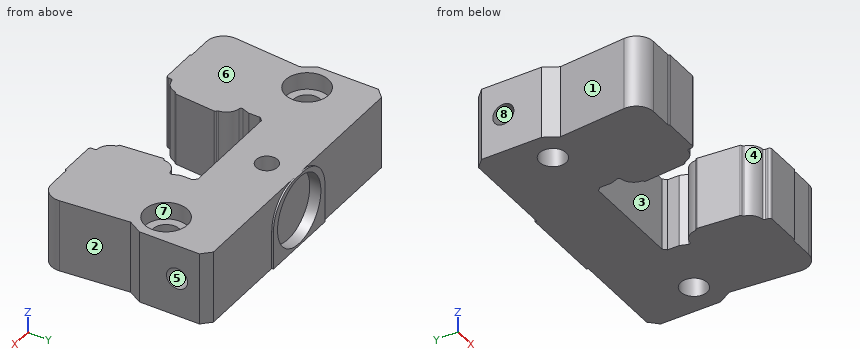
```python
from build123d import *

# Parameters (mm, degrees)
EXTRUDE1_DEPTH                          = 4.25
CBORE_FOR_M5_HEX_HEAD_BOLT2_D           = 3.1
CBORE_FOR_M5_HEX_HEAD_BOLT2_CBORE_D     = 5
CBORE_FOR_M5_HEX_HEAD_BOLT2_CBORE_DEPTH = 2
F_2_5_2_5_DIAMETER_HOLE1_D              = 2.5
F_2_5_2_5_DIAMETER_HOLE1_DEPTH          = 6
F_2_5_2_5_DIAMETER_HOLE1_TIP            = 0.751075774
SKETCH13_R                              = 4
EXTRUDE3_DEPTH                          = 0.2
CUT_EXTRUDE2_START                      = -1.3
SKETCH15_R                              = 4
CUT_EXTRUDE2_DEPTH                      = 1.3
FILLET1_R                               = 0.3
SKETCH16_W                              = 4.5
SKETCH16_H                              = 1.23


with BuildPart() as part:
    # Sketch1 → Extrude1 (new, symmetric)
    with BuildSketch(Plane.XY):
        with BuildLine():
            Line((4.92550995, -3.000896773), (5.340282634, -7.741770244))
            ThreePointArc((5.340282634, -7.741770244), (5.387571197, -7.845597639), (5.489639003, -7.896573115))
            ThreePointArc((5.489639003, -7.896573115), (5.583252131, -7.939368417), (5.635340188, -8.028147299))
            ThreePointArc((5.635340188, -8.028147299), (6.141739158, -8.88598399), (7.051010463, -9.292861611))
            ThreePointArc((7.051010463, -9.292861611), (7.196097182, -9.367838396), (7.25433228, -9.520417385))
            Line((7.25433228, -9.520417385), (7.25433228, -10.089549749))
            Line((7.25433228, -10.089549749), (11.66333313, -10.10000765))
            Line((11.66333313, -10.10000765), (11.81333313, -9.95000765))
            Line((11.81333313, -9.95000765), (14.47525163, -9.95000765))
            ThreePointArc((14.47525163, -9.95000765), (15.889465188, -9.36422121), (16.475251623, -7.95000765))
            ThreePointArc((16.475251623, -7.95000765), (16.473348066, -7.862768875), (16.467641019, -7.775696164))
            Line((16.467641019, -7.775696164), (15.777924964, 0.107794413))
            Line((15.777924964, 0.107794413), (16.697189707, 1.700007653))
            Line((16.697189707, 1.700007653), (16.697189707, 8.700007649))
            Line((16.697189707, 8.700007649), (15.697189707, 9.70000765))
            Line((15.697189707, 9.70000765), (-15.302810298, 9.70000765))
            Line((-15.302810298, 9.70000765), (-16.302810293, 8.700007655))
            Line((-16.302810293, 8.700007655), (-16.302810293, 1.70000765))
            Line((-16.302810293, 1.70000765), (-15.383545551, 0.107794412))
            Line((-15.383545551, 0.107794412), (-16.073261605, -7.775696165))
            ThreePointArc((-16.073261605, -7.775696165), (-15.555426882, -9.301188065), (-14.080872208, -9.95000765))
            Line((-14.080872208, -9.95000765), (-11.418953708, -9.95000765))
            Line((-11.418953708, -9.95000765), (-11.268953705, -10.10000765))
            Line((-11.268953705, -10.10000765), (-6.85995286, -10.089549753))
            Line((-6.85995286, -10.089549753), (-6.85995286, -9.520417385))
            ThreePointArc((-6.85995286, -9.520417385), (-6.801717763, -9.367838396), (-6.656631044, -9.292861611))
            ThreePointArc((-6.656631044, -9.292861611), (-5.747359739, -8.885983989), (-5.240960769, -8.028147299))
            ThreePointArc((-5.240960769, -8.028147299), (-5.188872711, -7.939368417), (-5.095259583, -7.896573115))
            ThreePointArc((-5.095259583, -7.896573115), (-4.993191778, -7.845597639), (-4.945903214, -7.741770244))
            Line((-4.945903214, -7.741770244), (-4.531130531, -3.000896773))
            ThreePointArc((-4.531130531, -3.000896773), (-4.530642578, -2.993452056), (-4.530479824, -2.985993141))
            ThreePointArc((-4.530479824, -2.985993141), (-4.563077813, -2.885564642), (-4.648443372, -2.823425817))
            ThreePointArc((-4.648443372, -2.823425817), (-4.731098063, -2.76492056), (-4.766166593, -2.669921291))
            ThreePointArc((-4.766166593, -2.669921291), (-5.198040021, -1.644927498), (-6.18433448, -1.130777545))
            ThreePointArc((-6.18433448, -1.130777545), (-6.349566009, -1.022272522), (-6.368749921, -0.825532146))
            Line((-6.368749921, -0.825532146), (-6.070902174, -0.007202189))
            ThreePointArc((-6.070902174, -0.007202189), (-6.057367635, 0.043309401), (-6.05280996, 0.095403855))
            Line((-6.05280996, 0.095403855), (-6.05280996, 1.399955293))
            Line((-6.05280996, 1.399955293), (-5.652810289, 1.800007648))
            Line((-5.652810289, 1.800007648), (6.047189708, 1.800007648))
            Line((6.047189708, 1.800007648), (6.44718938, 1.399955292))
            Line((6.44718938, 1.399955292), (6.44718938, 0.095403855))
            ThreePointArc((6.44718938, 0.095403855), (6.451747054, 0.043309401), (6.465281594, -0.007202188))
            Line((6.465281594, -0.007202188), (6.763129341, -0.825532146))
            ThreePointArc((6.763129341, -0.825532146), (6.773460706, -0.864089327), (6.77693973, -0.903854759))
            ThreePointArc((6.77693973, -0.903854759), (6.720404632, -1.054509523), (6.578713899, -1.130777545))
            ThreePointArc((6.578713899, -1.130777545), (5.59241944, -1.644927498), (5.160546013, -2.669921291))
            ThreePointArc((5.160546013, -2.669921291), (5.125477483, -2.76492056), (5.042822792, -2.823425817))
            ThreePointArc((5.042822792, -2.823425817), (4.953208331, -2.891697239), (4.92550995, -3.000896773))
        make_face()
    extrude(amount=EXTRUDE1_DEPTH, both=True)

    # CBORE for M5 Hex Head Bolt2 (through all)
    with Locations(Plane(origin=(-12.802810293, 2.596389855, 4.25), x_dir=(1, 0, 0), z_dir=(0, 0, 1))):
        with Locations((0, 0), (26, 0)):
            CounterBoreHole(CBORE_FOR_M5_HEX_HEAD_BOLT2_D / 2, CBORE_FOR_M5_HEX_HEAD_BOLT2_CBORE_D / 2, CBORE_FOR_M5_HEX_HEAD_BOLT2_CBORE_DEPTH)

    # Ø2.5 (2.5) Diameter Hole1
    with Locations(Plane(origin=(0.197189707, 6.127234967, 4.25), x_dir=(1, 0, 0), z_dir=(0, 0, 1))):
        with Locations((0, 0)):
            Hole(F_2_5_2_5_DIAMETER_HOLE1_D / 2, depth=F_2_5_2_5_DIAMETER_HOLE1_DEPTH)
            with Locations((0, 0, -(F_2_5_2_5_DIAMETER_HOLE1_DEPTH + F_2_5_2_5_DIAMETER_HOLE1_TIP / 2))):  # 118° drill point
                Cone(0, F_2_5_2_5_DIAMETER_HOLE1_D / 2, F_2_5_2_5_DIAMETER_HOLE1_TIP, mode=Mode.SUBTRACT)

    # Sketch13 → Extrude3 (add)
    with BuildSketch(Plane(origin=(0, 9.70000765, 0), x_dir=(1, 0, 0), z_dir=(0, 1, 0))):
        with BuildLine():
            Line((-4.552810293, 4.25), (-4.552810293, -0.25))
            ThreePointArc((-4.552810293, -0.25), (-3.381237418, -3.078427125), (-0.552810293, -4.25))
            Line((-0.552810293, -4.25), (0.947189707, -4.25))
            ThreePointArc((0.947189707, -4.25), (3.775616832, -3.078427125), (4.947189707, -0.25))
            Line((4.947189707, -0.25), (4.947189707, 4.25))
            Line((4.947189707, 4.25), (-4.552810293, 4.25))
        make_face()
        with Locations(Location((0.197189707, 0, 0), (0, 0, 270))):
            Circle(SKETCH13_R, mode=Mode.SUBTRACT)
    extrude(amount=EXTRUDE3_DEPTH)

    # Sketch15 → Cut-Extrude2 (cut)
    with BuildSketch(Plane(origin=(0, 9.90000765, 0), x_dir=(1, 0, 0), z_dir=(0, 1, 0)).offset(CUT_EXTRUDE2_START)):
        with Locations(Location((0.197189707, 0, 0), (0, 0, 270))):
            Circle(SKETCH15_R)
    extrude(amount=CUT_EXTRUDE2_DEPTH, mode=Mode.SUBTRACT)

    # Fillet1
    fillet1_edges = [part.edges().sort_by_distance(p)[0] for p in [
        (-6.85995286, -10.089549753, 0),
        (7.25433228, -10.089549749, 0),
    ]]
    fillet(fillet1_edges, radius=FILLET1_R)

    # Sketch16 → Cut-Revolve1 (revolve, cut)
    with BuildSketch(Plane(origin=(0.014534484, 6.127668215, 0), x_dir=(0.9999971869535607, -0.0023719369649562337, 0), z_dir=(-0.0023719369649562337, -0.9999971869535607, 0)), mode=Mode.PRIVATE) as cut_revolve1_sk:
        with Locations((14.443110426, 0.865)):
            Rectangle(SKETCH16_W, SKETCH16_H)
        with Locations((-14.073400302, 0.865)):
            Rectangle(SKETCH16_W, SKETCH16_H)
    revolve(cut_revolve1_sk.sketch.rotate(Axis((-24.587443164, 6.186022719, 0.25), (0.9999971869535605, -0.002371936964956225, 0)), 90), axis=Axis((-24.587443164, 6.186022719, 0.25), (0.9999971869535605, -0.002371936964956225, 0)), mode=Mode.SUBTRACT)


solid = part.part
```
Part model, mm, in its own coordinate system. Face numbers are marked on the shaded views. A direction names the side the tool comes from. Round coordinates to 2 decimals unless told otherwise and drop trailing zeros. Loops run counter-clockwise (first coordinate to the right, second up) from the corner with the lowest first, then second, coordinate; pieces in that order, holes last. Notation, with made-up numbers: (14.5, -31) -> (71.5, -31) arc R20 cw to (71.5, -5) -> close; hole circle Ø10 at (-10, -13). An arc over 180 degrees is marked (long way). Use a Markdown table: item, result.
1) Pull direction Z, two halves, no side cores. Call the marked faces 5, 6, 7 and 8: pulls with the +Z half, pulls with the -Z half, needs draft (parallel to the pull), parting line crosses it, or undercut.
The answers:
| item | result |
|---|---|
| face 5 | undercut |
| face 6 | pulls with the +Z half |
| face 7 | needs draft |
| face 8 | undercut |
2) Drop flat-ended pins along their axis: pin 1 Ø4 at (x, y) = (13.2, 2.6) entering from +Z; pin 2 Ø1.5 at (x, z) = (13.5, -1.5) entering from +Y; pin 3 Ø6 at (x, y) = (-12.8, 2.6) entering from -Z; pin 4 Ø5 at (y, z) = (-4.5, -0.5) entering from +X. Give the stop position or say it passes through.
The answers:
| item | result |
|---|---|
| pin 1 | stops at z = 2.25 |
| pin 2 | stops at y = 9.7 |
| pin 3 | stops at z = -4.25 |
| pin 4 | stops at x = 16.4 |
3) Tool access for the marked faces 1, 2, 3 and 4: list every direction of +Z, -Z, +X, -X, +Y, -Y with a clear straight run to the whole face (end or side of a thin tool).
The answers:
| item | result |
|---|---|
| face 1 | +Z, -Z, -X |
| face 2 | +Z, -Z, +X |
| face 3 | +Z, -Z |
| face 4 | +Z, -Z, -Y |
4) Cut at B-B, the plane y = -5.75. List the corners of the cut face in (x, z).
The answers:
| item | result |
|---|---|
| outline | (-15.9, -4.25) -> (-4.77, -4.25) -> (-4.77, 4.25) -> (-15.9, 4.25) -> close; (5.17, -4.25) -> (16.29, -4.25) -> (16.29, 4.25) -> (5.17, 4.25) -> close |
5) Cut at A-A, the plane y = 0.5. List the corners of the cut face in (x, z).
The answers:
| item | result |
|---|---|
| outline | (-15.61, -4.25) -> (-6.05, -4.25) -> (-6.05, 4.25) -> (-11.44, 4.25) -> (-11.44, 2.25) -> (-14.16, 2.25) -> (-14.16, 4.25) -> (-15.61, 4.25) -> close; (6.45, -4.25) -> (16, -4.25) -> (16, 4.25) -> (14.56, 4.25) -> (14.56, 2.25) -> (11.84, 2.25) -> (11.84, 4.25) -> (6.45, 4.25) -> close |
6) Cut at C-C, the plane z = 3.25. State how many separate pieces and enclosed holes the cut face has, and give its area (3 significant figures).
The answers:
| item | result |
|---|---|
| separate pieces | 1 |
| enclosed holes | 3 |
| area | 456 mm2 |
7) Probe line 1 (X direction, y = 2, z = -0.5); line 2 (Y direction, x = -4, z = 0.75); line 3 (X direction, y = -6.75, z = -0.5). List the from-to ranges inside material, lowest first. Write a range as [from, to].
The answers:
| item | result |
|---|---|
| line 1 | x = [-16.3, -14.23], [-11.37, 11.77], [14.63, 16.7] |
| line 2 | y = [1.8, 9.9] |
| line 3 | x = [-15.98, -4.86], [5.25, 16.38] |
